from build123d import *

# Parameters (mm, degrees)
SKETCH1_R           = 3.375
BOSS_EXTRUDE1_DEPTH = 1.65
SKETCH2_R           = 1.5
BOSS_EXTRUDE2_DEPTH = 8.35
CHAMFER1_SIZE       = 0.3
CUT_EXTRUDE1_DEPTH  = 2
CHAMFER2_SIZE       = 1.65


with BuildPart() as part:
    # Sketch1 → Boss-Extrude1 (new body)
    with BuildSketch(Plane.XY):
        Circle(SKETCH1_R)
    extrude(amount=BOSS_EXTRUDE1_DEPTH)

    # Sketch2 → Boss-Extrude2 (add)
    with BuildSketch(Plane(origin=(0, 0, 0), x_dir=(-1, 0, 0), z_dir=(0, 0, -1))):
        with Locations(Location((0, 0, 0), (0, 0, 180))):
            Circle(SKETCH2_R)
    extrude(amount=BOSS_EXTRUDE2_DEPTH)

    # Chamfer1
    chamfer1_edges = [part.edges().sort_by_distance(p)[0] for p in [
        (-1.5, 0, -8.35),
    ]]
    chamfer(chamfer1_edges, length=CHAMFER1_SIZE)

    # Sketch3 → Cut-Extrude1 (cut)
    with BuildSketch(Plane.XY.offset(1.65)):
        Polygon((0, 1.154700538), (-1, 0.577350269), (-1, -0.577350269), (0, -1.154700538), (1, -0.577350269), (1, 0.577350269), align=None)
    extrude(amount=-CUT_EXTRUDE1_DEPTH, mode=Mode.SUBTRACT)

    # Chamfer2
    chamfer2_edges = [part.edges().sort_by_distance(p)[0] for p in [
        (-3.375, 0, 0),
    ]]
    chamfer(chamfer2_edges, length=CHAMFER2_SIZE - 0.0001)  # a hair under: the kernel refuses the full size


solid = part.part
Work out the finished part from the listing and answer in its coordinate system (mm). A direction names the side the tool comes from. Give positions to 0.01 mm unless a question says otherwise; leave off trailing zeros. Order: outer loops, then holes, each group sorted by start corner. A loop starts at its lowest first (then second) coordinate and runs counter-clockwise, first axis right, second up. Notation, with made-up numbers: (-32.75, 82.5) -> (24.25, 82.5) arc R27 ccw to (24.25, 109.5) -> close; hole circle Ø10 at (82, 85.25). An arc over 180 degrees is marked (long way). Answer as a JSON object with one key per item and string values. Group by question number.
1. Section B-B on z = -2.25 is taken. Determine the outline of the cut face in (x, y), plus the area to 3 significant figures.
2. The mould has two halves that part along X. Classify faces 3 (the flat face through (1, 1, 1.65)), 4 (the flat face through (0.49, -0.87, 0.66)), 5 (the cylindrical face through (1.43, -0.45, -3.97)): released by +X, released by -X, zero draft, split by the parting line, or undercut.
3. A tool of negligible diameter and unlimited length cuts with its end or side. For faces 1 (the flat face through (0, 0, -8.35)), 2 (the flat face through (0.51, 0.86, 0.66)), from which of +Z, -Z, +X, -X, +Y, -Y can it reach the whole face along a straight path? Write none if from no direction.
4. Consider line 1 along Z through (x, y) = (1.5, 0.5); line 2 along Z through (x, y) = (-0.75, -0.5); line 3 along X through (y, z) = (0, 1.25). Determine where each line is inside the solid, lowest interval first. Write a range as [from, to].
5. Flat-ended cylindrical pins translate along their axes: pin 1 Ø3 at (y, z) = (-0.5, -3) entering from +X; pin 2 Ø1.5 at (x, z) = (0.5, -3) entering from -Y. Find the tip coordinate at first contact, or state that the pin passes through.
Result sheet:
{
 "1": {"outline": "circle Ø3 at (0, 0)", "area": "7.07 mm^2"},
 "2": {"face 3": "zero draft", "face 4": "undercut", "face 5": "split by the parting line"},
 "3": {"face 1": "-Z, +X, -X, +Y, -Y", "face 2": "+Z"},
 "4": {"line 1": "z = [0, 1.65]", "line 2": "z = [-8.35, -0.35]", "line 3": "x = [-2.98, -1], [1, 2.98]"},
 "5": {"pin 1": "stops at x = 1.5", "pin 2": "stops at y = -1.5"}
}
